Build history of the part. All positions in model axes, mm. Face numbers are marked on the shaded views. A direction names the side the tool comes from. Coordinates: 2 decimals unless noted, no trailing zeros. Write each loop counter-clockwise with the first axis right and the second up, starting at its lowest first coordinate (ties: lowest second). Pieces come first, ordered by that corner, then holes.
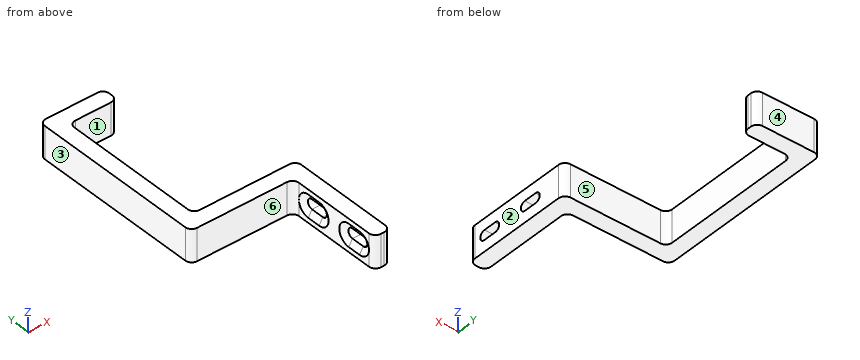
```python
from build123d import *

# Parameters (mm, degrees)
BOSS_EXTRUDE1_DEPTH     = 10
CUT_EXTRUDE1_DEPTH      = 93.303846074
CUT_EXTRUDE1_DEPTH_BACK = 93.303846074
CHAMFER2_SIZE           = 2
CHAMFER2_SIZE2          = 1.154700538
FILLET1_R               = 2


with BuildPart() as part:
    # Sketch1 → Boss-Extrude1 (new body)
    with BuildSketch(Plane.XY):
        Polygon((-14.5, 81), (-29.5, 81), (-29.5, 35), (2.5, 35), (2.5, 0), (-2.5, 0), (-2.5, 30), (-34.5, 30), (-34.5, 86), (-14.5, 86), align=None)
    extrude(amount=BOSS_EXTRUDE1_DEPTH)

    # Sketch3 → Cut-Extrude1 (cut, two sides: drawn at the far end of the back side and taken through both)
    with BuildSketch(Plane.ZY.offset(2.5).offset(-CUT_EXTRUDE1_DEPTH_BACK)):
        with BuildLine():
            Line((6.5, 24.5), (6.5, 20.5))
            ThreePointArc((6.5, 20.5), (5, 19), (3.5, 20.5))
            Line((3.5, 20.5), (3.5, 24.5))
            ThreePointArc((3.5, 24.5), (5, 26), (6.5, 24.5))
        make_face()
        with BuildLine():
            Line((6.5, 5.5), (6.5, 9.5))
            ThreePointArc((6.5, 9.5), (5, 11), (3.5, 9.5))
            Line((3.5, 9.5), (3.5, 5.5))
            ThreePointArc((3.5, 5.5), (5, 4), (6.5, 5.5))
        make_face()
    extrude(amount=CUT_EXTRUDE1_DEPTH + CUT_EXTRUDE1_DEPTH_BACK, mode=Mode.SUBTRACT)

    # Chamfer2
    chamfer2_edges = [part.edges().sort_by_distance(p)[0] for p in [
        (-2.5, 26, 5),
        (-2.5, 22.5, 6.5),
        (-2.5, 19, 5),
        (-2.5, 22.5, 3.5),
        (-2.5, 4, 5),
        (-2.5, 7.5, 3.5),
        (-2.5, 11, 5),
        (-2.5, 7.5, 6.5),
    ]]
    chamfer2_side = [part.faces().sort_by_distance(p)[0] for p in [
        (-2.5, 15, 5),
    ]]
    chamfer(chamfer2_edges, length=CHAMFER2_SIZE, length2=CHAMFER2_SIZE2, reference=chamfer2_side[0])

    # Fillet1
    fillet1_edges = [part.edges().sort_by_distance(p)[0] for p in [
        (-29.5, 81, 5),
        (-29.5, 35, 5),
        (2.5, 35, 5),
        (2.5, 0, 5),
        (-2.5, 0, 5),
        (-2.5, 30, 5),
        (-34.5, 30, 5),
        (-34.5, 86, 5),
        (-14.5, 86, 5),
        (-14.5, 81, 5),
    ]]
    fillet(fillet1_edges, radius=FILLET1_R - 0.0001)  # a hair under: the kernel refuses the full size


solid = part.part
```
1. Probe line 1 along Y through (x, z) = (-26.5, 8); line 2 along X through (y, z) = (76, 5.25); line 3 along Y through (x, z) = (-31, 7.25). List the from-to ranges inside material, lowest first.
Computed values:
line 1: y = 30 to 35, 81 to 86
line 2: x = -34.5 to -29.5
line 3: y = 30 to 86
2. Saw through at B-B on z = 5. State how many separate pieces and enclosed holes the cut face has, plus the area to 3 significant figures.
Computed values:
separate pieces: 3
enclosed holes: 0
area: 587 mm2
3. Saw through at C-C on y = 60. List the corners of the cut face in (x, z).
Computed values:
outline: (-34.5, 0) - (-29.5, 0) - (-29.5, 10) - (-34.5, 10) - close
4. Saw through at A-A on x = -21. List the corners of the cut face in (y, z).
Computed values:
outline: (30, 0) - (35, 0) - (35, 10) - (30, 10) - close; (81, 0) - (86, 0) - (86, 10) - (81, 10) - close
5. Saw through at D-D on x = -12.5. List the corners of the cut face in (y, z).
Computed values:
outline: (30, 0) - (35, 0) - (35, 10) - (30, 10) - close
6. 3-axis set-ups, long thin cutter, end or side, ignore diameter. For the marked faces 1 and 2: which of +Z, -Z, +X, -X, +Y, -Y reach the whole face in a straight line?
Computed values:
face 1: +Z, -Z, +X
face 2: +Z, -Z, +X, +Y, -Y
7. Flat gauge pins, fed straight in: pin 1 (2 mm diameter, centred on x = -13, z = 1.5, fed in from -Y); pin 2 (3 mm diameter, centred on y = 61.5, z = 2.5, fed in from +X); pin 3 (0.8 mm diameter, centred on y = 83.5, z = 7, fed in from +X). Where does each tip first touch, or does it go through?
Computed values:
pin 1: stops at y = 30
pin 2: stops at x = -29.5
pin 3: stops at x = -14.5
8. Mould opens along Y. For the marked faces 3, 4, 5 and 6 say: +Y half, -Y half, draft (parallel to the pull), parting line (faces both ways), or undercut.
Computed values:
face 3: draft
face 4: +Y half
face 5: undercut
face 6: -Y half
